Job drawing, mm, ordinate dimensions from the low corner. One solid piece. A direction names the side the tool comes from. Give positions to 0.01 mm unless a question says otherwise; leave off trailing zeros. Write each loop counter-clockwise with the first axis right and the second up, starting at its lowest first coordinate (ties: lowest second). Pieces come first, ordered by that corner, then holes. Notation, with made-up numbers: (27.5, -10.75) - (40.5, -10.75) arc R32 ccw to (40.5, 25.25) - close; hole circle Ø4 at (88.5, -20). An arc over 180 degrees is marked (long way). Answer in a Markdown table with one row per item. Add a question column.
1. Pull direction Y, two halves, no side cores. Call the marked faces 4, 5 and 6: released by +Y, released by -Y, zero draft, split by the parting line, or undercut.
2. Band-saw the part on D-D on x = 22.5. Write the cut outline in (y, z), plus the area to 3 significant figures.
3. Band-saw the part on C-C on z = 4.5. Write the cut outline in (x, y), plus the area to 3 significant figures.
4. Band-saw the part on A-A on x = 40. Write the cut outline in (y, z).
5. Drop flat-ended pins along their axis: pin 1 Ø4 at (x, z) = (19, 3.5) entering from +Y; pin 2 Ø4 at (y, z) = (24, 1) entering from +X; pin 3 Ø2 at (x, z) = (39, 4.5) entering from -Y. Give the stop position or say it passes through.
6. Band-saw the part on B-B on y = 13.5. Write the cut outline in (x, z), plus the area to 3 significant figures.
7. Which spindle directions (+Z, -Z, +X, -X, +Y, -Y) get a long thin tool onto all of the face, cutting with end or side? Do the marked faces 1, 2 and 3. Say none if no direction does.
8. Probe line 1 along Y through (x, z) = (5, 3.5); line 2 along Y through (x, z) = (22.5, 3.25); line 3 along X through (y, z) = (11.75, 2). List the from-to ranges inside material, lowest first.
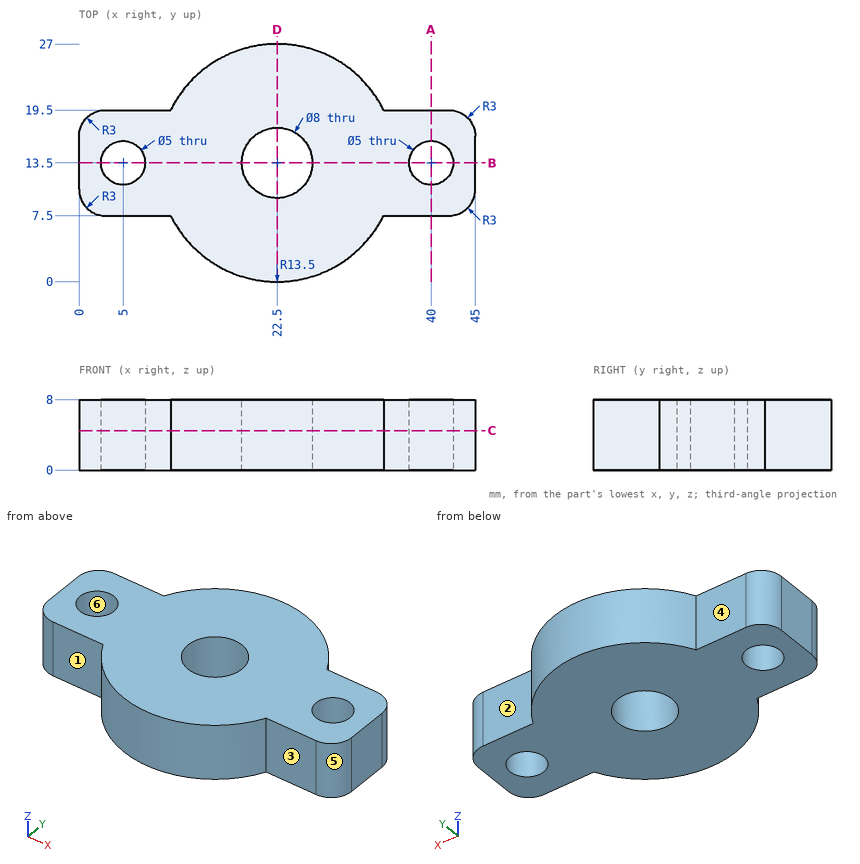
Values:
| question | item | result |
|---|---|---|
| 1 | face 4 | released by +Y |
| 1 | face 5 | released by -Y |
| 1 | face 6 | undercut |
| 2 | outline | (0, 0) - (9.5, 0) - (9.5, 8) - (0, 8) - close; (17.5, 0) - (27, 0) - (27, 8) - (17.5, 8) - close |
| 2 | area | 152 mm² |
| 3 | outline | (0, 10.5) arc R3 ccw to (3, 7.5) - (10.41, 7.5) arc R13.5 ccw to (34.59, 7.5) - (42, 7.5) arc R3 ccw to (45, 10.5) - (45, 16.5) arc R3 ccw to (42, 19.5) - (34.59, 19.5) arc R13.5 ccw to (10.41, 19.5) - (3, 19.5) arc R3 ccw to (0, 16.5) - close; hole circle Ø5 at (5, 13.5); hole circle Ø8 at (22.5, 13.5); hole circle Ø5 at (40, 13.5) |
| 3 | area | 702 mm² |
| 4 | outline | (7.5, 0) - (11, 0) - (11, 8) - (7.5, 8) - close; (16, 0) - (19.5, 0) - (19.5, 8) - (16, 8) - close |
| 5 | pin 1 | stops at y = 26.92 |
| 5 | pin 2 | stops at x = 32.99 |
| 5 | pin 3 | stops at y = 7.5 |
| 6 | outline | (0, 0) - (2.5, 0) - (2.5, 8) - (0, 8) - close; (7.5, 0) - (18.5, 0) - (18.5, 8) - (7.5, 8) - close; (26.5, 0) - (37.5, 0) - (37.5, 8) - (26.5, 8) - close; (42.5, 0) - (45, 0) - (45, 8) - (42.5, 8) - close |
| 6 | area | 216 mm² |
| 7 | face 1 | +Z, -Z, -X, -Y |
| 7 | face 2 | +Z, -Z, +X, +Y |
| 7 | face 3 | +Z, -Z, +X, -Y |
| 8 | line 1 | y = 7.5 to 11, 16 to 19.5 |
| 8 | line 2 | y = 0 to 9.5, 17.5 to 27 |
| 8 | line 3 | x = 0 to 3.21, 6.79 to 18.9, 26.1 to 38.21, 41.79 to 45 |
